```python
from build123d import *

# Parameters (mm, degrees)
EXTRUDE_1_DEPTH = 2
FILLET_1_R      = 2


with BuildPart() as part:
    # 草图1 → 凸台-拉伸1 (new body)
    with BuildSketch(Plane.XY):
        Polygon((81.505044408, -5.402721296), (76.505044408, -5.402721296), (76.505044408, 3.597278862), (72.505044408, 3.597278862), (72.505044408, 2.097278862), (69.305044408, 2.097278862), (69.305044408, 3.597278862), (66.105044408, 3.597278862), (66.105044408, 7.597278862), (69.305044408, 7.597278862), (69.305044408, 9.097278862), (72.505044408, 9.097278862), (72.505044408, 7.597278862), (76.505044408, 7.597278862), (76.505044408, 16.59727902), (81.505044408, 16.59727902), (81.505044408, 24.59727902), (76.505044688, 24.595607728), (66.105044408, 24.595607728), (42.505044408, 8.595607728), (32.535817857, 8.595607728), (-85.094955033, 24.595607728), (-95.494955312, 24.595607728), (-100.494955033, 24.59727902), (-100.494955033, 16.59727902), (-95.494955033, 16.59727902), (-95.494955033, 7.597278862), (-91.494955033, 7.597278862), (-91.494955033, 9.097278862), (-88.294955033, 9.097278862), (-88.294955033, 7.597278862), (-85.094955033, 7.597278862), (-85.094955033, 3.597278862), (-88.294955033, 3.597278862), (-88.294955033, 2.097278862), (-91.494955033, 2.097278862), (-91.494955033, 3.597278862), (-95.494955033, 3.597278862), (-95.494955033, -5.402721296), (-100.494955033, -5.402721296), (-100.494955033, -13.402721296), (-95.494955312, -13.401050004), (76.505044688, -13.401050004), (81.505044408, -13.402721296), align=None)
    extrude(amount=EXTRUDE_1_DEPTH)

    # 圆角1
    fillet_1_edges = [part.edges().sort_by_distance(p)[0] for p in [
        (42.505044408, 8.595607728, 1),
        (66.105044408, 24.595607728, 1),
        (81.505044408, 24.59727902, 1),
        (81.505044408, 16.59727902, 1),
        (81.505044408, -5.402721296, 1),
        (81.505044408, -13.402721296, 1),
        (-100.494955033, -13.402721296, 1),
        (-100.494955033, -5.402721296, 1),
        (-100.494955033, 16.59727902, 1),
        (-100.494955033, 24.59727902, 1),
    ]]
    fillet(fillet_1_edges, radius=FILLET_1_R)


solid = part.part
```
Build history of the part. All positions in model axes, mm. A direction names the side the tool comes from. Round coordinates to 2 decimals unless told otherwise and drop trailing zeros. Write each loop counter-clockwise with the first axis right and the second up, starting at its lowest first coordinate (ties: lowest second). Pieces come first, ordered by that corner, then holes.
1) Band-saw the part on B-B, the plane x = 30. List the corners of the cut face in (y, z).
2) Band-saw the part on A-A, the plane y = -2. List the corners of the cut face in (x, z), and give its area (3 significant figures).
3) Drill centre lines: probe 1 along Y at (x, z) = (68, 1.15); probe 2 along Y at (x, z) = (-88.5, 1.7); probe 3 along X at (y, z) = (-4, 1.5). Where is each one in solid material? Low to high.
4) Pin check, flat tips, straight feed: pin 1 (0.8 mm diameter, centred on y = 3, z = 1.5, fed in from +X); pin 2 (10 mm diameter, centred on x = 45, y = 13.5, fed in from -Z); pin 3 (1.2 mm diameter, centred on y = 3, z = 1.5, fed in from -X). Stop position of each tip, or through.
5) Mould opens along X. For faces 3 (the flat face through (-25.456, 16.484, 0.986)), 4 (the flat face through (-11, 2, 0)) say: +X half, -X half, draft (parallel to the pull), parting line (faces both ways), or undercut.
6) 3-axis set-ups, long thin cutter, end or side, ignore diameter. For faces 1 (the flat face through (54.46, 16.7, 0.99)), 2 (the flat face through (-11, 2, 2)): which of +Z, -Z, +X, -X, +Y, -Y reach the whole face in a straight line?
Ans:
1. outline: (-13.4, 0) - (8.94, 0) - (8.94, 2) - (-13.4, 2) - close
2. outline: (-95.49, 0) - (76.51, 0) - (76.51, 2) - (-95.49, 2) - close
2. area: 344 mm2
3. probe 1: y = -13.4 to 3.6, 7.6 to 24.6
3. probe 2: y = -13.4 to 2.1, 9.1 to 24.6
3. probe 3: x = -95.49 to 76.51
4. pin 1: stops at x = 76.51
4. pin 2: stops at z = 0
4. pin 3: stops at x = -95.49
5. face 3: undercut
5. face 4: draft
6. face 1: +Z, -Z, +Y
6. face 2: +Z, +X, -X, +Y, -Y
